Geometry check sheet. Reference: the model listing, model coordinates, mm. A direction names the side the tool comes from. Coordinates: 2 decimals unless noted, no trailing zeros. Loops run counter-clockwise (first coordinate to the right, second up) from the corner with the lowest first, then second, coordinate; pieces in that order, holes last. Notation, with made-up numbers: (70.25, -27.5) - (116.25, -27.5) arc R36 ccw to (116.25, 7.5) - close; hole circle Ø7 at (-31.75, -5.75). An arc over 180 degrees is marked (long way). One line per item, written item: value.
Autodesk Inventor part; units mm, degrees
ref_plane "YZ Plane" through (0, 0, 0) normal (1, 0, 0) x (0, 1, 0)
ref_plane "XZ Plane" through (0, 0, 0) normal (0, 1, 0) x (-1, 0, 0)
ref_plane "XY Plane" through (0, 0, 0) normal (0, 0, 1) x (1, 0, 0)
sketch "스케치1" plane through (0, 0, 0) normal (0, 0, 1) x (1, 0, 0)
  circle A0 centre (0, 0) radius 10.8
  circle A1 centre (0, 0) radius 6
  circle A2 centre (0, -8) radius 1.05
  circle A3 centre (-5.6569, -5.6569) radius 1.05
  circle A4 centre (-8, 0) radius 1.05
  circle A5 centre (-5.6569, 5.6569) radius 1.05
  circle A6 centre (0, 8) radius 1.05
  circle A7 centre (5.6569, 5.6569) radius 1.05
  circle A8 centre (8, 0) radius 1.05
  circle A9 centre (5.6569, -5.6569) radius 1.05
  circle A10 centre (0, 0) radius 3.6
  circle A11 centre (0, 0) radius 3.6
  circle A12 centre (0, 0) radius 4
  line L0 (-4, 0) -> (4, 0)
  line L1 (4, 0) -> (4, -13.3653)
  line L2 (4, -13.3653) -> (-4, -13.3653)
  line L3 (-4, -13.3653) -> (-4, 0)
  line L4 (-10.8, 0) -> (10.8, 0)
  line L5 (10.8, 0) -> (10.8, 100)
  line L6 (10.8, 100) -> (-10.8, 100)
  line L7 (-10.8, 100) -> (-10.8, 0)
  line L8 (10.8, 100) -> (10.8, 94)
  line L9 (10.8, 94) -> (3.6, 94)
  line L10 (3.6, 94) -> (-3.6, 94)
  line L11 (-3.6, 94) -> (-10.8, 94)
  circle A13 centre (-3.6, 94) radius 1.35
  circle A14 centre (3.6, 94) radius 1.35
  point P0 (0, 0)
  point P1 (-3.6, 0)
  point P2 (3.6, 0)
  point P3 (-4, -10.0319)
  point P4 (4, -10.0319)
  dimension "d0" = 8
  dimension "d1" = 100
  dimension "d2" = 21.6
  dimension "d3" = 6
  dimension "d4" = 7.2
  dimension "d5" = 7.2
  dimension "d6" = 2.7
  dimension "d7" = 2.7
extrude "돌출1" add sketch "스케치1" along normal blind 6 contours L4 A8 A1 A4 A0 | A0 L1 A1 L4 A8 | A0 L7 L11 A13 L10 A14 L9 L5 | L4 A4 A1 L3 A0 | L9 A14 L10 A13 L11 L7 L6 L5 | L1 L4 A1 | A1 L4 L3 | L4 A12 A1
properties part number "_hand_adt_ver_2_" material "PMMA 플라스틱"
(1) Cross-section at C-C on z = 4.35. State how many separate pieces and enclosed holes the cut face has, and give its area (3 significant figures).
Reply:
separate pieces: 1
enclosed holes: 9
area: 2,200 mm2
(2) Cross-section at B-B on y = 94. Record the cut outline in (x, z).
Reply:
outline: (-10.8, 0) - (-4.95, 0) - (-4.95, 6) - (-10.8, 6) - close; (-2.25, 0) - (2.25, 0) - (2.25, 6) - (-2.25, 6) - close; (4.95, 0) - (10.8, 0) - (10.8, 6) - (4.95, 6) - close
(3) Material ranges on probe 1 along X at (y, z) = (94, 3.8); probe 2 along X at (y, z) = (0, 2.25); probe 3 along X at (y, z) = (6, 0.35), recorded low to high. Write a range as from..to.
Reply:
probe 1: -10.8..-4.95, -2.25..2.25, 4.95..10.8
probe 2: -10.8..-9.05, -6.95..-4, 4..6.95, 9.05..10.8
probe 3: -10.8..-6.65, -4.66..4.66, 6.65..10.8
(4) Cross-section at D-D on y = 8. Record the cut outline in (x, z).
Reply:
outline: (-10.8, 0) - (-1.05, 0) - (-1.05, 6) - (-10.8, 6) - close; (1.05, 0) - (10.8, 0) - (10.8, 6) - (1.05, 6) - close
(5) Go/stop test with flat-tipped pins: pin 1 Ø1.8 at (y, z) = (-5, 3) entering from +X; pin 2 Ø2.5 at (x, y) = (8, 0) entering from -Z; pin 3 Ø1.8 at (y, z) = (-7, 3) entering from -X. Record where each tip stops, or that it passes through.
Reply:
pin 1: x = 9.99
pin 2: z = 0
pin 3: x = -8.91
(6) Release check for a two-part mould opening along X. For faces 1 (the face through (0, 46, 6)), 2 (the face through (-4, -5, 3)), 3 (the face through (10.8, 49, 3)) record: pulls with the +X half, pulls with the -X half, needs draft (parallel to the pull), parting line crosses it, or undercut.
Reply:
face 1: needs draft
face 2: undercut
face 3: pulls with the +X half
(7) Access from +Z, -Z, +X, -X, +Y, -Y to the whole of each face (thin tool, end or side, straight path). Record for faces 4 (the face through (4, -5, 3)), 5 (the face through (4.883, -6.367, 2.958)).
Reply:
face 4: +Z, -Z, -Y
face 5: +Z, -Z
(8) Cross-section at A-A on x = 0. Record the cut outline in (y, z), and give its area (3 significant figures).
Reply:
outline: (4, 0) - (6.95, 0) - (6.95, 6) - (4, 6) - close; (9.05, 0) - (100, 0) - (100, 6) - (9.05, 6) - close
area: 563 mm2
